from build123d import *

# Parameters (mm, degrees)
BOSS_EXTRUDE1_DEPTH        = 1
BOSS_EXTRUDE1_DEPTH_BACK   = 3
SKETCH1_R                  = 0.4
BOSS_EXTRUDE1_2_DEPTH      = 1
BOSS_EXTRUDE1_2_DEPTH_BACK = 3


with BuildPart() as part:
    # Sketch1 → Boss-Extrude1 (new, two sides: drawn at the far end of the back side and taken through both)
    with BuildSketch(Plane(origin=(0, 0, 0), x_dir=(1, 0, 0), z_dir=(0, 1, 0)).offset(-BOSS_EXTRUDE1_DEPTH_BACK)):
        with Locations(Location((-2.5, 0, 0), (0, 0, 270))):
            Circle(SKETCH1_R)
    extrude(amount=BOSS_EXTRUDE1_DEPTH + BOSS_EXTRUDE1_DEPTH_BACK)



with BuildPart() as body_2:
    # Sketch1 → Boss-Extrude1 2 (new, two sides: drawn at the far end of the back side and taken through both)
    with BuildSketch(Plane(origin=(0, 0, 0), x_dir=(1, 0, 0), z_dir=(0, 1, 0)).offset(-BOSS_EXTRUDE1_2_DEPTH_BACK)):
        with Locations(Location((2.5, 0, 0), (0, 0, 90))):
            Circle(SKETCH1_R)
    extrude(amount=BOSS_EXTRUDE1_2_DEPTH + BOSS_EXTRUDE1_2_DEPTH_BACK)


with BuildPart() as part_1:
    add(part.part)

    add(body_2.part)  # Revolve1 merges body 2
    # Sketch3 → Revolve1 (revolve)
    with BuildSketch(Plane.XY):
        with BuildLine():
            Line((5, 0.5), (5, 0.75))
            ThreePointArc((5, 0.75), (4.933012702, 1), (4.75, 1.183012702))
            ThreePointArc((4.75, 1.183012702), (4.5, 1.616025404), (4.75, 2.049038106))
            ThreePointArc((4.75, 2.049038106), (4.933012702, 2.232050808), (5, 2.482050808))
            Line((5, 2.482050808), (5, 19.7))
            ThreePointArc((5, 19.7), (4.853553391, 20.053553391), (4.5, 20.2))
            Line((4.5, 20.2), (4, 20.2))
            Line((4, 20.2), (4, 20.1))
            Line((4, 20.1), (0, 20.1))
            Line((0, 20.1), (0, 0.1))
            Line((0, 0.1), (4, 0.1))
            Line((4, 0.1), (4, 0))
            Line((4, 0), (4.5, 0))
            ThreePointArc((4.5, 0), (4.853553391, 0.146446609), (5, 0.5))
        make_face()
    revolve(axis=Axis((0, 0.1, 0), (0, 1, 0)))


solid = part_1.part
Geometry check sheet. Reference: the model listing, model coordinates, mm. A direction names the side the tool comes from. Give positions to 0.01 mm unless a question says otherwise; leave off trailing zeros. Loops run counter-clockwise (first coordinate to the right, second up) from the corner with the lowest first, then second, coordinate; pieces in that order, holes last.
(1) Set-up check for faces 4 (the flat face through (-3, 20.2, 3)), 5 (the flat face through (0, 20.1, 0)): record each of +Z, -Z, +X, -X, +Y, -Y from which the full face is reachable in a straight line by a thin tool's end or side.
From the geometry:
face 4: +Z, -Z, +X, -X, +Y
face 5: +Y
(2) Section check B-B on y = 1.75. Record the cut outline in (x, z), then the cut area to 3 significant figures.
From the geometry:
outline: circle Ø9.04 at (0, 0)
area: 64.1 mm2
(3) Section check A-A on y = 12. Record the cut outline in (x, z).
From the geometry:
outline: circle Ø10 at (0, 0)
(4) Release check for a two-part mould opening along Z. For faces 1 (the flat face through (0, 0.1, 0)), 2 (the flat face through (3, 0, 3)), 3 (the cylindrical face through (-1.08, 11.21, 4.88)) record: released by +Z, released by -Z, zero draft, split by the parting line, or undercut.
From the geometry:
face 1: undercut
face 2: zero draft
face 3: split by the parting line
(5) Thickness scan on L1, parallel to Y at x = -3, z = 2.5; L2, parallel to Y at x = -2.75, z = 4; L3, parallel to Y at x = 2, z = 4.5. Record the ranges inside material, lowest first.
From the geometry:
L1: y = 0.1 to 20.1
L2: y = 0.15 to 1.1, 2.13 to 20.05
L3: y = 0.24 to 1.01, 2.22 to 19.96
(6) Depth check by flat-ended pin: pin 1 Ø4 at (x, z) = (0, 1) entering from +Y; pin 2 Ø5 at (y, z) = (3.5, 4) entering from +X; pin 3 Ø6 at (x, z) = (-1.5, -3) entering from +Y; pin 4 Ø3 at (x, z) = (2, -3) entering from -Y. Enter the tip coordinate at first touch or a pass-through.
From the geometry:
pin 1: stops at y = 20.1
pin 2: stops at x = 4.77
pin 3: stops at y = 20.2
pin 4: stops at y = 0
